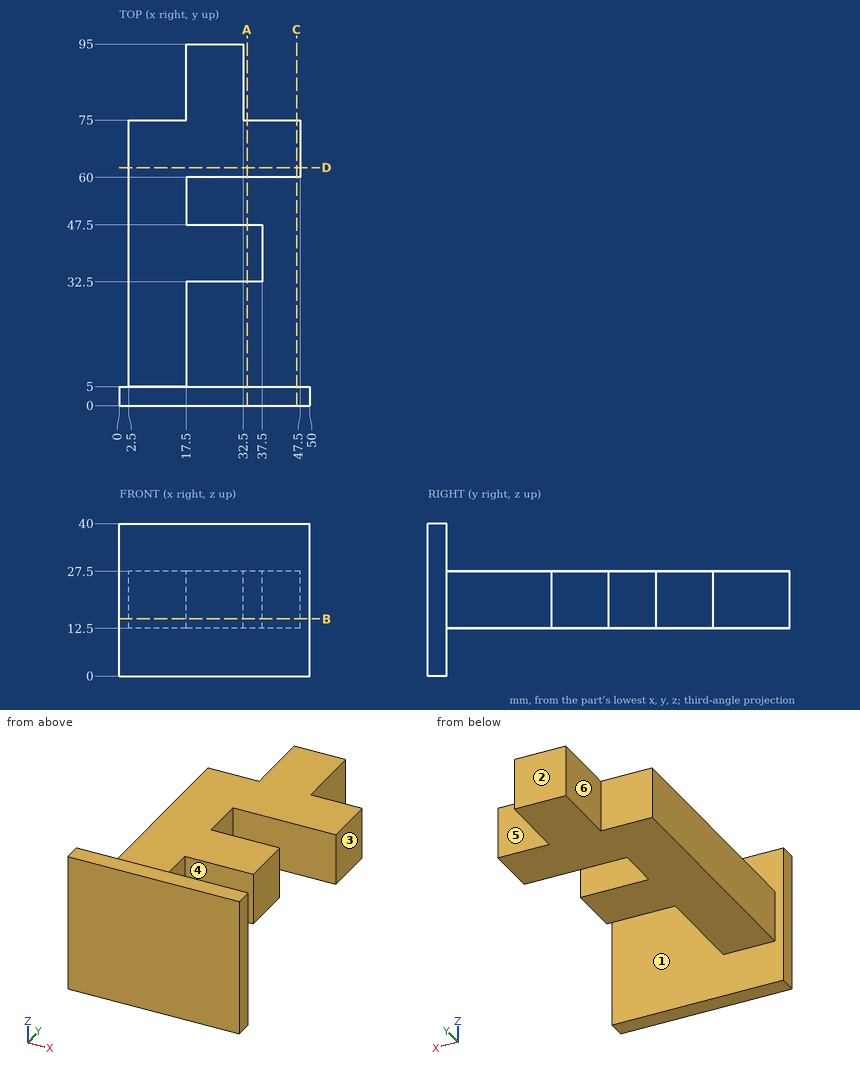
Could you check a few things on this drawing? It's one solid part, dimensions in mm from its lowest x, y, z. A direction names the side the tool comes from. Give positions to 0.01 mm unless a question says otherwise; leave off trailing zeros. Loops run counter-clockwise (first coordinate to the right, second up) from the corner with the lowest first, then second, coordinate; pieces in that order, holes last. Notation, with made-up numbers: M 87,85.5 L 96,85.5 A13 cw 96,94.5 Z; hole C 79,78.25 d3. An arc over 180 degrees is marked long. Answer as a JSON object with one key per item and string values.
Q1. Suppose I cut it at B-B, the plane z = 15. List the corners of the cut face in (x, y) for me.
Values found:
{"outline": "M 0,0 L 50,0 L 50,5 L 17.5,5 L 17.5,32.5 L 37.5,32.5 L 37.5,47.5 L 17.5,47.5 L 17.5,60 L 47.5,60 L 47.5,75 L 32.5,75 L 32.5,95 L 17.5,95 L 17.5,75 L 2.5,75 L 2.5,5 L 0,5 Z"}
Q2. For the marked faces 4, 5 and 6, which set-ups out of +Z, -Z, +X, -X, +Y, -Y let a thin tool reach every point of the face, with its end or its side?
Values found:
{"face 4": "+Z, -Z, +X", "face 5": "+Z, -Z, +X, +Y", "face 6": "+Z, -Z, -X, +Y"}
Q3. For P1, Ø4.5, axis at x = 39.5, z = 23.5, coming from the +Y side; P2, Ø10, axis at x = 8.5, y = 33.5, coming from the -Z side; P3, Ø4.5, axis at y = 40.5, z = 21.5, coming from the +X side; P4, Ø6, axis at y = 47.5, z = 32, coming from the +X side, each with a flat end and sliding along its axis, tell me the tip position at first contact or that it passes through.
Values found:
{"P1": "stops at y = 75", "P2": "stops at z = 12.5", "P3": "stops at x = 37.5", "P4": "passes through"}
Q4. Suppose I cut it at D-D, the plane y = 62.5. List the corners of the cut face in (x, z) for me, plus the area to 3 significant figures.
Values found:
{"outline": "M 2.5,12.5 L 47.5,12.5 L 47.5,27.5 L 2.5,27.5 Z", "area": "675 mm²"}
Q5. Suppose I cut it at A-A, the plane x = 33.5. List the corners of the cut face in (y, z) for me, plus the area to 3 significant figures.
Values found:
{"outline": "M 0,0 L 5,0 L 5,40 L 0,40 Z; M 32.5,12.5 L 47.5,12.5 L 47.5,27.5 L 32.5,27.5 Z; M 60,12.5 L 75,12.5 L 75,27.5 L 60,27.5 Z", "area": "650 mm²"}
Q6. If I drill on probe 1 along Y at (x, z) = (37, 14); probe 2 along Y at (x, z) = (38, 14); probe 3 along Y at (x, z) = (25.5, 12), over which ranges is the centre line in solid material (lowest first)? Write a range as [from, to].
Values found:
{"probe 1": "y = [0, 5], [32.5, 47.5], [60, 75]", "probe 2": "y = [0, 5], [60, 75]", "probe 3": "y = [0, 5]"}
Q7. Suppose I cut it at C-C, the plane x = 46.5. List the corners of the cut face in (y, z) for me, plus the area to 3 significant figures.
Values found:
{"outline": "M 0,0 L 5,0 L 5,40 L 0,40 Z; M 60,12.5 L 75,12.5 L 75,27.5 L 60,27.5 Z", "area": "425 mm²"}
Q8. If we mould it in two halves opening along Y, with no side actions, what happens to the marked faces 1, 2 and 3? For each: pulls with the +Y half, pulls with the -Y half, needs draft (parallel to the pull), parting line crosses it, or undercut.
Values found:
{"face 1": "undercut", "face 2": "pulls with the +Y half", "face 3": "needs draft"}
